Could you check a few things on this drawing? It's one solid part, dimensions in mm from its lowest x, y, z. Round coordinates to 2 decimals unless told otherwise and drop trailing zeros. Loops run counter-clockwise (first coordinate to the right, second up) from the corner with the lowest first, then second, coordinate; pieces in that order, holes last. Notation, with made-up numbers: (33, 38.25) -> (84, 38.25) arc R6 ccw to (84, 45.25) -> close; hole circle Ø6 at (49.5, 46). An arc over 180 degrees is marked (long way). Use one line per item in the form item = value. Start each with the question number.
Item 1: Thinking about a two-plate mould opening in Y: for the marked faces 1, 2, 3 and 4, which applies, released by +Y, released by -Y, zero draft, split by the parting line, or undercut?
Item 2: I'm going to push a flat-ended pin straight in: pin 1 Ø9 at (y, z) = (27.25, 10) entering from -X. Where does the tip first touch, or does it pass through?
Item 3: If we section it at A-A (y = 10): Write out the boundary of the cut face in (x, z).
Item 4: If we section it at C-C (x = 3.35): State how many separate pieces and enclosed holes the cut face has, then the cut area to 3 significant figures.
Item 5: If I drill on L1, parallel to Y at x = 2.45, z = 10; L2, parallel to Y at x = 0.6, z = 8.5 (1 decimal); L3, parallel to Z at x = 3.4, y = 8.5 (1 decimal), over which ranges is the centre line in solid material (lowest first)? Write a range as [from, to].
Item 6: If we section it at B-B (z = 10): Write out the boundary of the cut face in (x, y).
Item 7: If we section it at D-D (y = 27.25): Write out the boundary of the cut face in (x, z).
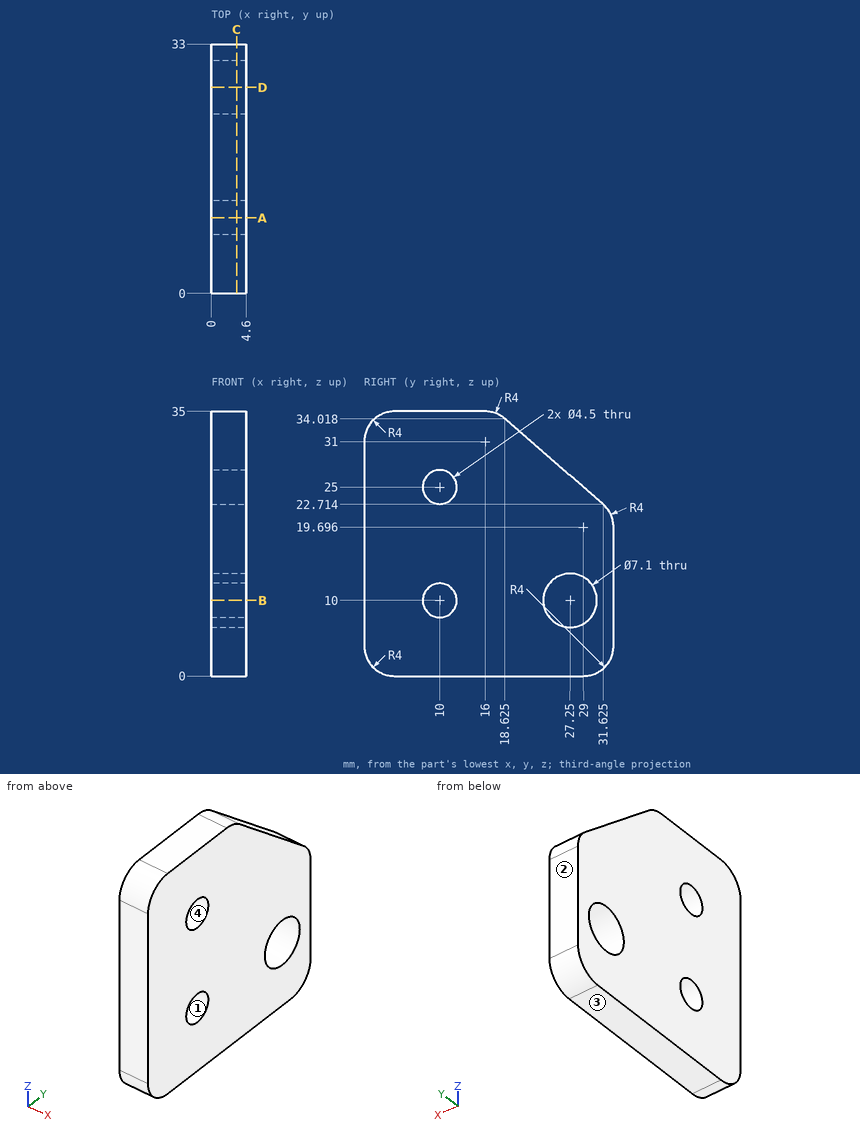
Values found:
q1.face_1 = undercut
q1.face_2 = released by +Y
q1.face_3 = zero draft
q1.face_4 = undercut
q2.pin_1 = 0
q3.outline = (0, 0) -> (4.6, 0) -> (4.6, 7.75) -> (0, 7.75) -> close; (0, 12.25) -> (4.6, 12.25) -> (4.6, 22.75) -> (0, 22.75) -> close; (0, 27.25) -> (4.6, 27.25) -> (4.6, 35) -> (0, 35) -> close
q4.separate_pieces = 1
q4.enclosed_holes = 3
q4.area = 968 mm2
q5.L1 = [0, 7.75], [12.25, 23.7], [30.8, 33]
q5.L2 = [0, 8.3], [11.7, 24], [30.5, 33]
q5.L3 = [0, 8.3], [11.7, 23.3], [26.7, 35]
q6.outline = (0, 0) -> (4.6, 0) -> (4.6, 7.75) -> (0, 7.75) -> close; (0, 12.25) -> (4.6, 12.25) -> (4.6, 23.7) -> (0, 23.7) -> close; (0, 30.8) -> (4.6, 30.8) -> (4.6, 33) -> (0, 33) -> close
q7.outline = (0, 0) -> (4.6, 0) -> (4.6, 6.45) -> (0, 6.45) -> close; (0, 13.55) -> (4.6, 13.55) -> (4.6, 26.52) -> (0, 26.52) -> close
